Could you check a few things on this model? Use its own coordinates, in mm. A direction names the side the tool comes from. Give positions to 0.01 mm unless a question says otherwise; leave off trailing zeros. Write each loop counter-clockwise with the first axis right and the second up, starting at its lowest first coordinate (ties: lowest second). Pieces come first, ordered by that corner, then holes. Notation, with made-up numbers: M 78.25,88 L 131.25,88 A19 ccw 131.25,125 Z; hole C -8,18.5 d10. An arc over 180 degrees is marked long. Use one line per item in the form item = value.
Autodesk Inventor part; units mm, degrees
ref_plane "YZ Plane" through (0, 0, 0) normal (1, 0, 0) x (0, 1, 0)
ref_plane "XZ Plane" through (0, 0, 0) normal (0, 1, 0) x (-1, 0, 0)
ref_plane "XY Plane" through (0, 0, 0) normal (0, 0, 1) x (1, 0, 0)
sketch "Sketch1" plane through (0, 0, 0) normal (0, 0, 1) x (1, 0, 0)
  line L0 (-7.83, 0) -> (7.83, 0)
  line L1 (7.83, 0) -> (7.83, 2.3813)
  line L2 (7.83, 2.3813) -> (3.092, 2.3813)
  line L3 (3.092, 2.3813) -> (3.092, 3.4544)
  line L4 (3.092, 3.4544) -> (2.33, 3.4544)
  line L5 (2.33, 3.4544) -> (2.33, 2.3813)
  line L6 (2.33, 2.3813) -> (-6.052, 2.3812)
  line L7 (-6.052, 2.3812) -> (-7.83, 1.905)
  line L8 (-7.83, 1.905) -> (-7.83, 0)
  point P0 (0, 0)
  point P1 (0, 0)
  dimension "d0" = 4.7625
  dimension "d1" = 10.16
  dimension "d2" = 6.9088
  dimension "d3" = 1.778
  dimension "d4" = 3.81
  dimension "d5" = 0.762
  dimension "d6" = 5.5
  dimension "d7" = 4.738
revolve "Revolution1" add sketch "Sketch1" angle 360 about axis through (-7.83, 0, 0) along (1, 0, 0)
sketch "Sketch2" plane through (0, 0, 0) normal (0, 1, 0) x (-1, 0, 0)
  line L0 (-3.092, 2.3812) -> (-3.092, -2.3812)
  line L1 (-3.092, 0) -> (-7.83, 0) construction
  circle A0 centre (-5.461, 0) radius 1
  line L2 (-7.83, 2.3812) -> (-7.83, -2.3812)
  point P0 (0, 0)
  point P1 (-7.33, 2.3812)
  point P2 (-7.33, -2.3812)
  dimension "d12" = 2
extrude "Extrusion1" cut sketch "Sketch2" along normal through all both and the other way through all
chamfer "Chamfer2" distance 0.3 angle 45 4 edges at (7.83, -2.3812, 0) (5.4611, 2.1611, 1) (5.4609, 2.1611, -1) (6.461, -2.3812, -0.003)
sketch "Sketch3" plane through (0, 0, 0) normal (0, 0, 1) x (1, 0, 0)
  line L0 (-6.052, 2.3812) -> (2.33, 2.3812)
  line L1 (-7.83, -1.905) -> (-7.83, 1.905)
  arc A0 (-2.7246, 2.1654) -> (-3.9946, 2.1654) centre (-3.3596, 2.1654) ccw
  line L2 (-3.9946, 2.1654) -> (-2.7246, 2.1654)
  line L3 (-6.052, -2.3812) -> (2.33, -2.3812)
  line L4 (2.33, -3.4544) -> (2.33, 3.4544)
  point P0 (0, 0)
  point P1 (-3.3596, 2.8004)
  point P2 (-2.7624, 2.3812)
  dimension "d18" = 4.4704
  dimension "d20" = 5.1816
  dimension "d21" = 1.27
  dimension "d22" = 5.0924
revolve "Revolution2" add sketch "Sketch3" angle 360 about axis through (-3.9946, 2.1654, 0) along (1, 0, 0)
properties part number "Pin_RBF" material "Stainless Steel"
1) Thinking about a two-plate mould opening in Z: for faces 3 (the flat face through (7.83, 0, 0)), 4 (the cylindrical face through (-1.92, 1.1, 2.11)), 5 (the cylindrical face through (4.507, -0.029, -0.3)), which applies, released by +Z, released by -Z, zero draft, split by the parting line, or undercut?
Checked values:
face_3 = zero draft
face_4 = split by the parting line
face_5 = undercut
2) I want a section at A-A, the plane y = 0. Please give me the cut outline in (x, z) (3 decimals).
Checked values:
outline = M -7.83,-1.905 L -6.052,-2.381 L 2.33,-2.381 L 2.33,-3.454 L 3.092,-3.454 L 3.092,-2.381 L 7.53,-2.381 L 7.83,-2.081 L 7.83,2.081 L 7.53,2.381 L 3.092,2.381 L 3.092,3.454 L 2.33,3.454 L 2.33,2.381 L -6.052,2.381 L -7.83,1.905 Z; hole C 5.461,0 d2
3) If I drill on L1, parallel to X at y = 0.9, z = 0; L2, parallel to X at y = -2.25, z = 1.5; L3, parallel to Z at x = -2.75, y = 2, over which ranges is the centre line in solid material (lowest first)?
Checked values:
L1 = -7.83 to 4.46, 6.46 to 7.83
L2 = 2.33 to 3.09
L3 = -1.29 to 1.29
4) For faces 1 (the flat face through (-7.83, 0, 0)), 2 (the cylindrical face through (5.28, -1.755, -1.609)), which set-ups out of +Z, -Z, +X, -X, +Y, -Y let a thin tool reach every point of the face, with its end or its side?
Checked values:
face_1 = +Z, -Z, -X, +Y, -Y
face_2 = +X
5) I want a section at C-C, the plane y = 3. Please give me the cut outline in (x, z), plus the area to 3 significant figures.
Checked values:
outline = M 2.33,-1.71 L 3.09,-1.71 L 3.09,1.71 L 2.33,1.71 Z
area = 2.61 mm2
6) I want a section at D-D, the plane z = 3.25. Please give me the cut outline in (x, y).
Checked values:
outline = M 2.33,-1.17 L 3.09,-1.17 L 3.09,1.17 L 2.33,1.17 Z
7) For pin 1 Ø3 at (x, y) = (2, 1.5) entering from +Z; pin 2 Ø2.5 at (x, z) = (5.461, 0) entering from -Y; pin 3 Ø4 at (x, z) = (-4, 2) entering from +Y; pin 4 Ø3 at (x, z) = (5.5, 1) entering from +Y, each with a flat end and sliding along its axis, tell me the tip position at first contact or that it passes through.
Checked values:
pin_1 = 3.45
pin_2 = -2.33
pin_3 = 2.79
pin_4 = 2.38
8) I want a section at B-B, the plane x = 3.5. Please give me the cut outline in (y, z).
Checked values:
outline = C 0,0 d4.76
